Build history of the part. All positions in model axes, mm. A direction names the side the tool comes from. Coordinates: 2 decimals unless noted, no trailing zeros. Loops run counter-clockwise (first coordinate to the right, second up) from the corner with the lowest first, then second, coordinate; pieces in that order, holes last. Notation, with made-up numbers: (11, 47.25) -> (55, 47.25) arc R25 cw to (55, 59.25) -> close; hole circle Ø8 at (23, 8.5). An arc over 180 degrees is marked (long way). One line per item, written item: value. Start each with the question number.
```python
from build123d import *

# Parameters (mm, degrees)
SKETCH_1_R          = 9.5
EXTRUDE_1_DEPTH     = 8
SKETCH_3_R          = 2
CUT_EXTRUDE_2_DEPTH = 8
SKETCH_4_R          = 5
CUT_EXTRUDE_3_DEPTH = 8
SKETCH_5_W          = 12
SKETCH_5_H          = 120
CUT_EXTRUDE_4_DEPTH = 10
EXTRUDE_2_DEPTH     = 8


with BuildPart() as part:
    # 草图1 → 凸台-拉伸1 (new body)
    with BuildSketch(Plane.XY):
        with BuildLine():
            Line((-10, 76.819660113), (-10, -76.819660113))
            ThreePointArc((-10, -76.819660113), (0, -103), (10, -76.819660113))
            Line((10, -76.819660113), (10, 76.819660113))
            ThreePointArc((10, 76.819660113), (0, 103), (-10, 76.819660113))
        make_face()
        with Locations((0, -88)):
            Circle(SKETCH_1_R, mode=Mode.SUBTRACT)
    extrude(amount=EXTRUDE_1_DEPTH)

    # 草图3 → 切除-拉伸2 (cut)
    with BuildSketch(Plane.XY.offset(8)):
        with Locations((0, 98)):
            Circle(SKETCH_3_R)
        with Locations((10, 88)):
            Circle(SKETCH_3_R)
        with Locations((0, 78)):
            Circle(SKETCH_3_R)
        with Locations((-10, 88)):
            Circle(SKETCH_3_R)
        with Locations((7.071067812, 95.071067812)):
            Circle(SKETCH_3_R)
        with Locations((7.071067812, 80.928932188)):
            Circle(SKETCH_3_R)
        with Locations((-7.071067812, 80.928932188)):
            Circle(SKETCH_3_R)
        with Locations((-7.071067812, 95.071067812)):
            Circle(SKETCH_3_R)
    extrude(amount=-CUT_EXTRUDE_2_DEPTH, mode=Mode.SUBTRACT)

    # 草图4 → 切除-拉伸3 (cut)
    with BuildSketch(Plane.XY.offset(8)):
        with Locations((0, 88)):
            Circle(SKETCH_4_R)
    extrude(amount=-CUT_EXTRUDE_3_DEPTH, mode=Mode.SUBTRACT)

    # 草图5 → 切除-拉伸4 (cut)
    with BuildSketch(Plane.XY.offset(8)):
        with BuildLine():
            ThreePointArc((-6, 60), (0, 66), (6, 60))
            Line((6, 60), (-6, 60))
        make_face()
        Rectangle(SKETCH_5_W, SKETCH_5_H)
        with BuildLine():
            Line((-6, -60), (6, -60))
            ThreePointArc((6, -60), (0, -66), (-6, -60))
        make_face()
    extrude(amount=-CUT_EXTRUDE_4_DEPTH, mode=Mode.SUBTRACT)

    # 草图6 → 凸台-拉伸2 (add)
    with BuildSketch(Plane.XY.offset(8)):
        with BuildLine():
            Line((-6, 10), (-6, -10))
            ThreePointArc((-6, -10), (0, -4), (6, -10))
            Line((6, -10), (6, 10))
            ThreePointArc((6, 10), (0, 4), (-6, 10))
        make_face()
    extrude(amount=-EXTRUDE_2_DEPTH)


solid = part.part
```
Item 1: Probe probe 1 along X at (y, z) = (19.5, 5.25); probe 2 along Y at (x, z) = (2.25, 5.5); probe 3 along Y at (x, z) = (8.75, 1.25). List the from-to ranges inside material, lowest first.
Item 2: Band-saw the part on C-C, the plane y = 88. List the corners of the cut face in (x, z).
Item 3: Band-saw the part on B-B, the plane x = -0.25. List the corners of the cut face in (y, z), and give its area (3 significant figures).
Item 4: Tool access for faces 1 (the face through (0, -4, 4)), 2 (the face through (-10, 1, 4)), 3 (the face through (10, -1, 4)): list every direction of +Z, -Z, +X, -X, +Y, -Y with a clear straight run to the whole face (end or side of a thin tool).
Item 5: Two-plate mould, pull along Y, no slides. Class faces 4 (the face through (0, 1, 8)), 5 (the face through (6.64, 93.12, 4.06)): +Y half, -Y half, draft (parallel to the pull), parting line (faces both ways), or undercut.
Item 6: Band-saw the part on D-D, the plane z = 1.5. Count the separate pieces of the cut face and the enclosed holes in it, and give its area (3 significant figures).
Item 7: Band-saw the part on A-A, the plane y = 13. List the corners of the cut face in (x, z), and give its area (3 significant figures).
Item 8: Drop flat-ended pins along their axis: pin 1 Ø3 at (y, z) = (42, 3.5) entering from +X; pin 2 Ø1 at (y, z) = (-81.5, 3.5) entering from -X; pin 3 Ø3 at (y, z) = (-11.5, 2) entering from -X; pin 4 Ø3.5 at (x, y) = (7.07, 80.93) entering from -Z. Give the stop position or say it passes through.
Worked out:
1. probe 1: x = -10 to -6, 6 to 10
1. probe 2: y = -102.83 to -97.23, -78.77 to -65.56, -4.44 to 4.44, 65.56 to 83.53, 92.47 to 102.83
1. probe 3: y = -100.18 to -91.7, -84.3 to 79.84, 82.02 to 86.44, 89.56 to 93.98, 96.16 to 100.18
2. outline: (-15, 0) -> (-12, 0) -> (-12, 8) -> (-15, 8) -> close; (-8, 0) -> (-5, 0) -> (-5, 8) -> (-8, 8) -> close; (5, 0) -> (8, 0) -> (8, 8) -> (5, 8) -> close; (12, 0) -> (15, 0) -> (15, 8) -> (12, 8) -> close
3. outline: (-103, 0) -> (-97.5, 0) -> (-97.5, 8) -> (-103, 8) -> close; (-78.5, 0) -> (-65.99, 0) -> (-65.99, 8) -> (-78.5, 8) -> close; (-4.01, 0) -> (4.01, 0) -> (4.01, 8) -> (-4.01, 8) -> close; (65.99, 0) -> (76.02, 0) -> (76.02, 8) -> (65.99, 8) -> close; (79.98, 0) -> (83.01, 0) -> (83.01, 8) -> (79.98, 8) -> close; (92.99, 0) -> (96.02, 0) -> (96.02, 8) -> (92.99, 8) -> close; (99.98, 0) -> (103, 0) -> (103, 8) -> (99.98, 8) -> close
3. area: 361 mm²
4. face 1: +Z, -Z
4. face 2: +Z, -Z, -X
4. face 3: +Z, -Z, +X
5. face 4: draft
5. face 5: undercut
6. separate pieces: 1
6. enclosed holes: 12
6. area: 2,490 mm²
7. outline: (-10, 0) -> (-6, 0) -> (-6, 8) -> (-10, 8) -> close; (6, 0) -> (10, 0) -> (10, 8) -> (6, 8) -> close
7. area: 64.0 mm²
8. pin 1: stops at x = 10
8. pin 2: stops at x = -13.75
8. pin 3: stops at x = -10
8. pin 4: passes through
